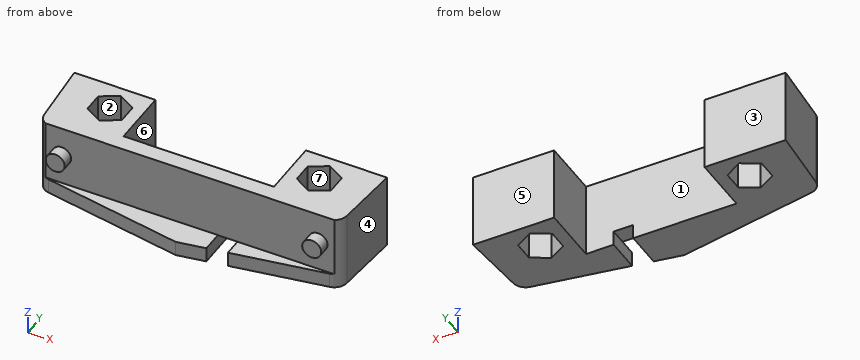
```python
from build123d import *

# Parameters (mm, degrees)
SKETCH1_W           = 9
SKETCH1_H           = 9
BOSS_EXTRUDE1_DEPTH = 11.5
SKETCH2_W           = 45.5
SKETCH2_H           = 9.25
CUT_EXTRUDE1_DEPTH  = 4
SKETCH3_R           = 1.45
BOSS_EXTRUDE2_DEPTH = 1.8
CUT_EXTRUDE2_REACH  = 32.72
SKETCH4_W           = 3
SKETCH4_H           = 2.25


with BuildPart() as part:
    # Sketch1 → Boss-Extrude1 (new body)
    # profile 1 of 4: a face of its own
    with BuildSketch(Plane.XY):
        with BuildLine():
            Line((-20.5, -76.5), (-23.900700066, -76.5))
            Line((-23.900700066, -76.5), (-23.121499045, -86.400687699))
            ThreePointArc((-23.121499045, -86.400687699), (-22.608100633, -87.588503122), (-21.474960733, -88.213385013))
            Line((-21.474960733, -88.213385013), (0, -92))
            Line((0, -92), (21.474960733, -88.213385013))
            ThreePointArc((21.474960733, -88.213385013), (22.608100633, -87.588503122), (23.121499045, -86.400687699))
            Line((23.121499045, -86.400687699), (23.900700066, -76.5))
            Line((23.900700066, -76.5), (20.5, -76.5))
            Line((20.5, -76.5), (20.5, -85.5))
            Line((20.5, -85.5), (11.5, -85.5))
            Line((11.5, -85.5), (-11.5, -85.5))
            Line((-11.5, -85.5), (-20.5, -85.5))
            Line((-20.5, -85.5), (-20.5, -76.5))
        make_face()
    # profile 2 of 4: a face of its own
    with BuildSketch(Plane.XY):
        with BuildLine():
            Line((-20.5, -76.5), (-23.900700066, -76.5))
            Line((-23.900700066, -76.5), (-23.121499045, -86.400687699))
            ThreePointArc((-23.121499045, -86.400687699), (-22.608100633, -87.588503122), (-21.474960733, -88.213385013))
            Line((-21.474960733, -88.213385013), (0, -92))
            Line((0, -92), (21.474960733, -88.213385013))
            ThreePointArc((21.474960733, -88.213385013), (22.608100633, -87.588503122), (23.121499045, -86.400687699))
            Line((23.121499045, -86.400687699), (23.900700066, -76.5))
            Line((23.900700066, -76.5), (20.5, -76.5))
            Line((20.5, -76.5), (20.5, -85.5))
            Line((20.5, -85.5), (11.5, -85.5))
            Line((11.5, -85.5), (-11.5, -85.5))
            Line((-11.5, -85.5), (-20.5, -85.5))
            Line((-20.5, -85.5), (-20.5, -76.5))
        make_face()
    # profile 3 of 4: a face of its own
    with BuildSketch(Plane.XY):
        with Locations((16, -81)):
            Rectangle(SKETCH1_W, SKETCH1_H)
        Polygon((18.625, -82.515544457), (16, -84.031088913), (13.375, -82.515544457), (13.375, -79.484455543), (16, -77.968911087), (18.625, -79.484455543), align=None, mode=Mode.SUBTRACT)
    # profile 4 of 4: a face of its own
    with BuildSketch(Plane.XY):
        with Locations((-16, -81)):
            Rectangle(SKETCH1_W, SKETCH1_H)
        Polygon((-13.375, -82.515544457), (-16, -84.031088913), (-18.625, -82.515544457), (-18.625, -79.484455543), (-16, -77.968911087), (-13.375, -79.484455543), align=None, mode=Mode.SUBTRACT)
    extrude(amount=BOSS_EXTRUDE1_DEPTH)

    # Sketch2 → Cut-Extrude1 (cut)
    with BuildSketch(Plane(origin=(0, -92, 0), x_dir=(1, 0, 0), z_dir=(0, 1, 0))):
        with Locations((0, -6.875)):
            Rectangle(SKETCH2_W, SKETCH2_H)
    extrude(amount=CUT_EXTRUDE1_DEPTH, mode=Mode.SUBTRACT)

    # Sketch3 → Boss-Extrude2 (add)
    with BuildSketch(Plane.XZ.offset(88)):
        with Locations(Location((-19.6, 6.875, 0), (0, 0, 270))):
            Circle(SKETCH3_R)
        with Locations(Location((19.6, 6.875, 0), (0, 0, 90))):
            Circle(SKETCH3_R)
    extrude(amount=BOSS_EXTRUDE2_DEPTH)

    # Sketch4 → Cut-Extrude2 (cut, up to next)
    with BuildSketch(Plane(origin=(0, -92, 0), x_dir=(1, 0, 0), z_dir=(0, 1, 0)), mode=Mode.PRIVATE) as cut_extrude2_sk1:
        with Locations((5.78456273, -1.125)):
            Rectangle(SKETCH4_W, SKETCH4_H)
    cut_extrude2_tool1 = extrude(cut_extrude2_sk1.sketch, amount=CUT_EXTRUDE2_REACH, mode=Mode.PRIVATE) & part.part
    add(cut_extrude2_tool1.solids().sort_by_distance((5.784563, -92, 1.125))[0], mode=Mode.SUBTRACT)


solid = part.part
```
Design review of the part built by this model. Coordinates are the model's own, in mm. Face numbers are marked on the shaded views. A direction names the side the tool comes from. Give positions to 0.01 mm unless a question says otherwise; leave off trailing zeros. Write each loop counter-clockwise with the first axis right and the second up, starting at its lowest first coordinate (ties: lowest second). Pieces come first, ordered by that corner, then holes.
(1) Mouldability with a two-part tool opening along Y and no side actions: class the marked faces 4, 5, 6 and 7 as +Y half, -Y half, draft (parallel to the pull), parting line (faces both ways), or undercut.
Checked values:
face 4: -Y half
face 5: +Y half
face 6: draft
face 7: undercut
(2) Tool access review of the marked faces 1, 2 and 3: name each direction out of +Z, -Z, +X, -X, +Y, -Y from which nothing blocks a thin tool from reaching the whole face with its end or side.
Checked values:
face 1: +Z, -Z, +Y
face 2: +Z, -Z
face 3: +Z, -Z, +X, -X, +Y
(3) Add section B-B (z = 8.75). Give the boundary of the cut face in (x, y) (1 decimal), and give its area (3 significant figures).
Checked values:
outline: (-23.9, -76.5) - (-23.1, -86.4) arc R2 ccw to (-22.1, -88) - (22.1, -88) arc R2 ccw to (23.1, -86.4) - (23.9, -76.5) - (11.5, -76.5) - (11.5, -85.5) - (-11.5, -85.5) - (-11.5, -76.5) - close; hole (-18.6, -82.5) - (-16, -84) - (-13.4, -82.5) - (-13.4, -79.5) - (-16, -78) - (-18.6, -79.5) - close; hole (13.4, -82.5) - (16, -84) - (18.6, -82.5) - (18.6, -79.5) - (16, -78) - (13.4, -79.5) - close
area: 284 mm2
(4) Clearance check with flat-ended pins moving along their axes: pin 1 Ø0.9 at (x, z) = (-19, 6.5) entering from -Y; pin 2 Ø0.9 at (y, z) = (-80.5, 8) entering from -X; pin 3 Ø0.7 at (y, z) = (-88, 0.5) entering from -X. State where each tip first meets the part, or that it passes through.
Checked values:
pin 1: stops at y = -89.8
pin 2: stops at x = -23.62
pin 3: stops at x = -22.55
(5) Add section A-A (z = 1.25). Give the boundary of the cut face in (x, y) (1 decimal), and give its area (3 significant figures).
Checked values:
outline: (-23.9, -76.5) - (-23.1, -86.4) arc R2 ccw to (-21.5, -88.2) - (0, -92) - (4.3, -91.2) - (4.3, -85.5) - (-11.5, -85.5) - (-11.5, -76.5) - close; (7.3, -90.7) - (21.5, -88.2) arc R2 ccw to (23.1, -86.4) - (23.9, -76.5) - (11.5, -76.5) - (11.5, -85.5) - (7.3, -85.5) - close; hole (-18.6, -82.5) - (-16, -84) - (-13.4, -82.5) - (-13.4, -79.5) - (-16, -78) - (-18.6, -79.5) - close; hole (13.4, -82.5) - (16, -84) - (18.6, -82.5) - (18.6, -79.5) - (16, -78) - (13.4, -79.5) - close
area: 358 mm2
(6) Add section C-C (y = -87.25). Give the boundary of the cut face in (x, z).
Checked values:
outline: (-22.86, 0) - (4.28, 0) - (4.28, 2.25) - (7.28, 2.25) - (7.28, 0) - (22.86, 0) - (22.86, 11.5) - (-22.86, 11.5) - close
(7) Wall thickness on line 1 along X through (y, z) = (-88.5, 6.75); line 2 along X through (y, z) = (-78.5, 3); line 3 along X through (y, z) = (-82.5, 6.75) (3 decimals): over which ranges is each line inside the solid? List them lowest first.
Checked values:
line 1: x = -21.04 to -18.16, 18.16 to 21.04
line 2: x = -23.74 to -16.92, -15.08 to -11.5, 11.5 to 15.08, 16.92 to 23.74
line 3: x = -23.428 to -18.625, -13.375 to -11.5, 11.5 to 13.375, 18.625 to 23.428
(8) Add section D-D (x = -7). Give the boundary of the cut face in (y, z), and give its area (3 significant figures).
Checked values:
outline: (-90.77, 0) - (-85.5, 0) - (-85.5, 11.5) - (-88, 11.5) - (-88, 2.25) - (-90.77, 2.25) - close
area: 35.0 mm2
